Part model, mm, in its own coordinate system. Coordinates: 2 decimals unless noted, no trailing zeros. Write each loop counter-clockwise with the first axis right and the second up, starting at its lowest first coordinate (ties: lowest second). Pieces come first, ordered by that corner, then holes. Notation, with made-up numbers: (80, 5) -> (104, 5) arc R11 cw to (104, 11) -> close; hole circle Ø1 at (58, 56). An arc over 180 degrees is marked (long way). Write item = value, one per line.
from build123d import *

# Parameters (mm, degrees)
BOSS_EXTRUDE1_DEPTH      = 2.54
SKETCH2_W                = 0.64
SKETCH2_H                = 0.64
BOSS_EXTRUDE2_DEPTH      = 6
BOSS_EXTRUDE2_DEPTH_BACK = 5.74


with BuildPart() as part:
    # Sketch1 → Boss-Extrude1 (new body)
    with BuildSketch(Plane(origin=(0, 0, 0), x_dir=(1, 0, 0), z_dir=(0, 1, 0))):
        with BuildLine():
            Line((-11.43, -1.016), (-11.43, 1.016))
            ThreePointArc((-11.43, 1.016), (-11.504394878, 1.195605122), (-11.684, 1.27))
            Line((-11.684, 1.27), (-13.716, 1.27))
            ThreePointArc((-13.716, 1.27), (-13.895605122, 1.195605122), (-13.97, 1.016))
            Line((-13.97, 1.016), (-13.97, -1.016))
            ThreePointArc((-13.97, -1.016), (-13.895605122, -1.195605122), (-13.716, -1.27))
            Line((-13.716, -1.27), (-11.684, -1.27))
            ThreePointArc((-11.684, -1.27), (-11.504394878, -1.195605122), (-11.43, -1.016))
        make_face()
        with BuildLine():
            Line((-8.89, -1.016), (-8.89, 1.016))
            ThreePointArc((-8.89, 1.016), (-8.964394878, 1.195605122), (-9.144, 1.27))
            Line((-9.144, 1.27), (-11.176, 1.27))
            ThreePointArc((-11.176, 1.27), (-11.355605122, 1.195605122), (-11.43, 1.016))
            Line((-11.43, 1.016), (-11.43, -1.016))
            ThreePointArc((-11.43, -1.016), (-11.355605122, -1.195605122), (-11.176, -1.27))
            Line((-11.176, -1.27), (-9.144, -1.27))
            ThreePointArc((-9.144, -1.27), (-8.964394878, -1.195605122), (-8.89, -1.016))
        make_face()
        with BuildLine():
            Line((-6.35, -1.016), (-6.35, 1.016))
            ThreePointArc((-6.35, 1.016), (-6.424394878, 1.195605122), (-6.604, 1.27))
            Line((-6.604, 1.27), (-8.636, 1.27))
            ThreePointArc((-8.636, 1.27), (-8.815605122, 1.195605122), (-8.89, 1.016))
            Line((-8.89, 1.016), (-8.89, -1.016))
            ThreePointArc((-8.89, -1.016), (-8.815605122, -1.195605122), (-8.636, -1.27))
            Line((-8.636, -1.27), (-6.604, -1.27))
            ThreePointArc((-6.604, -1.27), (-6.424394878, -1.195605122), (-6.35, -1.016))
        make_face()
        with BuildLine():
            Line((-3.81, -1.016), (-3.81, 1.016))
            ThreePointArc((-3.81, 1.016), (-3.884394878, 1.195605122), (-4.064, 1.27))
            Line((-4.064, 1.27), (-6.096, 1.27))
            ThreePointArc((-6.096, 1.27), (-6.275605122, 1.195605122), (-6.35, 1.016))
            Line((-6.35, 1.016), (-6.35, -1.016))
            ThreePointArc((-6.35, -1.016), (-6.275605122, -1.195605122), (-6.096, -1.27))
            Line((-6.096, -1.27), (-4.064, -1.27))
            ThreePointArc((-4.064, -1.27), (-3.884394878, -1.195605122), (-3.81, -1.016))
        make_face()
        with BuildLine():
            Line((-1.27, -1.016), (-1.27, 1.016))
            ThreePointArc((-1.27, 1.016), (-1.344394878, 1.195605122), (-1.524, 1.27))
            Line((-1.524, 1.27), (-3.556, 1.27))
            ThreePointArc((-3.556, 1.27), (-3.735605122, 1.195605122), (-3.81, 1.016))
            Line((-3.81, 1.016), (-3.81, -1.016))
            ThreePointArc((-3.81, -1.016), (-3.735605122, -1.195605122), (-3.556, -1.27))
            Line((-3.556, -1.27), (-1.524, -1.27))
            ThreePointArc((-1.524, -1.27), (-1.344394878, -1.195605122), (-1.27, -1.016))
        make_face()
        with BuildLine():
            Line((1.27, -1.016), (1.27, 1.016))
            ThreePointArc((1.27, 1.016), (1.195605122, 1.195605122), (1.016, 1.27))
            Line((1.016, 1.27), (-1.016, 1.27))
            ThreePointArc((-1.016, 1.27), (-1.195605122, 1.195605122), (-1.27, 1.016))
            Line((-1.27, 1.016), (-1.27, -1.016))
            ThreePointArc((-1.27, -1.016), (-1.195605122, -1.195605122), (-1.016, -1.27))
            Line((-1.016, -1.27), (1.016, -1.27))
            ThreePointArc((1.016, -1.27), (1.195605122, -1.195605122), (1.27, -1.016))
        make_face()
        with BuildLine():
            Line((3.81, -1.016), (3.81, 1.016))
            ThreePointArc((3.81, 1.016), (3.735605122, 1.195605122), (3.556, 1.27))
            Line((3.556, 1.27), (1.524, 1.27))
            ThreePointArc((1.524, 1.27), (1.344394878, 1.195605122), (1.27, 1.016))
            Line((1.27, 1.016), (1.27, -1.016))
            ThreePointArc((1.27, -1.016), (1.344394878, -1.195605122), (1.524, -1.27))
            Line((1.524, -1.27), (3.556, -1.27))
            ThreePointArc((3.556, -1.27), (3.735605122, -1.195605122), (3.81, -1.016))
        make_face()
        with BuildLine():
            Line((6.35, -1.016), (6.35, 1.016))
            ThreePointArc((6.35, 1.016), (6.275605122, 1.195605122), (6.096, 1.27))
            Line((6.096, 1.27), (4.064, 1.27))
            ThreePointArc((4.064, 1.27), (3.884394878, 1.195605122), (3.81, 1.016))
            Line((3.81, 1.016), (3.81, -1.016))
            ThreePointArc((3.81, -1.016), (3.884394878, -1.195605122), (4.064, -1.27))
            Line((4.064, -1.27), (6.096, -1.27))
            ThreePointArc((6.096, -1.27), (6.275605122, -1.195605122), (6.35, -1.016))
        make_face()
        with BuildLine():
            Line((8.89, -1.016), (8.89, 1.016))
            ThreePointArc((8.89, 1.016), (8.815605122, 1.195605122), (8.636, 1.27))
            Line((8.636, 1.27), (6.604, 1.27))
            ThreePointArc((6.604, 1.27), (6.424394878, 1.195605122), (6.35, 1.016))
            Line((6.35, 1.016), (6.35, -1.016))
            ThreePointArc((6.35, -1.016), (6.424394878, -1.195605122), (6.604, -1.27))
            Line((6.604, -1.27), (8.636, -1.27))
            ThreePointArc((8.636, -1.27), (8.815605122, -1.195605122), (8.89, -1.016))
        make_face()
        with BuildLine():
            Line((11.43, -1.016), (11.43, 1.016))
            ThreePointArc((11.43, 1.016), (11.355605122, 1.195605122), (11.176, 1.27))
            Line((11.176, 1.27), (9.144, 1.27))
            ThreePointArc((9.144, 1.27), (8.964394878, 1.195605122), (8.89, 1.016))
            Line((8.89, 1.016), (8.89, -1.016))
            ThreePointArc((8.89, -1.016), (8.964394878, -1.195605122), (9.144, -1.27))
            Line((9.144, -1.27), (11.176, -1.27))
            ThreePointArc((11.176, -1.27), (11.355605122, -1.195605122), (11.43, -1.016))
        make_face()
        with BuildLine():
            Line((13.97, -1.016), (13.97, 1.016))
            ThreePointArc((13.97, 1.016), (13.895605122, 1.195605122), (13.716, 1.27))
            Line((13.716, 1.27), (11.684, 1.27))
            ThreePointArc((11.684, 1.27), (11.504394878, 1.195605122), (11.43, 1.016))
            Line((11.43, 1.016), (11.43, -1.016))
            ThreePointArc((11.43, -1.016), (11.504394878, -1.195605122), (11.684, -1.27))
            Line((11.684, -1.27), (13.716, -1.27))
            ThreePointArc((13.716, -1.27), (13.895605122, -1.195605122), (13.97, -1.016))
        make_face()
    extrude(amount=BOSS_EXTRUDE1_DEPTH)

    # Sketch2 → Boss-Extrude2 (add, two sides)
    with BuildSketch(Plane(origin=(0, 2.54, 0), x_dir=(1, 0, 0), z_dir=(0, 1, 0))) as boss_extrude2_sk:
        with Locations((-12.7, 0)):
            Rectangle(SKETCH2_W, SKETCH2_H)
        with Locations((-10.16, 0)):
            Rectangle(SKETCH2_W, SKETCH2_H)
        with Locations((-7.62, 0)):
            Rectangle(SKETCH2_W, SKETCH2_H)
        with Locations((-5.08, 0)):
            Rectangle(SKETCH2_W, SKETCH2_H)
        with Locations((-2.54, 0)):
            Rectangle(SKETCH2_W, SKETCH2_H)
        Rectangle(SKETCH2_W, SKETCH2_H)
        with Locations((2.54, 0)):
            Rectangle(SKETCH2_W, SKETCH2_H)
        with Locations((5.08, 0)):
            Rectangle(SKETCH2_W, SKETCH2_H)
        with Locations((7.62, 0)):
            Rectangle(SKETCH2_W, SKETCH2_H)
        with Locations((10.16, 0)):
            Rectangle(SKETCH2_W, SKETCH2_H)
        with Locations((12.7, 0)):
            Rectangle(SKETCH2_W, SKETCH2_H)
    extrude(amount=BOSS_EXTRUDE2_DEPTH)
    extrude(boss_extrude2_sk.sketch, amount=-BOSS_EXTRUDE2_DEPTH_BACK)


solid = part.part
Q1. Saw through at A-A on y = 5. Count the separate pieces of the cut face and the enclosed holes in it, and give its area (3 significant figures).
Model answer:
separate_pieces = 11
enclosed_holes = 0
area = 4.51 mm²
Q2. Probe line 1 (Y direction, x = -2, z = 0.85); line 2 (Z direction, x = 0.25, y = 3.5). List the from-to ranges inside material, lowest first. Write a range as from..to.
Model answer:
line_1 = 0..2.54
line_2 = -0.32..0.32
Q3. Mould opens along X. For faces 1 (the face through (0, 0, -1)), 2 (the face through (13.97, 1, 0)), 3 (the face through (0, 2.54, -1)), 4 (the face through (8, 1, 1.27)) say: released by +X, released by -X, zero draft, split by the parting line, or undercut.
Model answer:
face_1 = undercut
face_2 = released by +X
face_3 = undercut
face_4 = zero draft
Q4. Pin check, flat tips, straight feed: pin 1 (0.7 mm diameter, centred on y = 5, z = 0, fed in from -X); pin 2 (0.5 mm diameter, centred on y = 7, z = 0, fed in from +X); pin 3 (0.5 mm diameter, centred on x = 0, y = 5, fed in from -Z). Stop position of each tip, or through.
Model answer:
pin_1 = -13.02
pin_2 = 13.02
pin_3 = -0.32
Q5. Saw through at B-B on x = 2.5. Give the cut face in (y, z), and give its area (3 significant figures).
Model answer:
outline = (-3.2, -0.32) -> (0, -0.32) -> (0, -1.27) -> (2.54, -1.27) -> (2.54, -0.32) -> (8.54, -0.32) -> (8.54, 0.32) -> (2.54, 0.32) -> (2.54, 1.27) -> (0, 1.27) -> (0, 0.32) -> (-3.2, 0.32) -> close
area = 12.3 mm²
Q6. Saw through at D-D on x = -10.75. Give the cut face in (y, z), and give its area (3 significant figures).
Model answer:
outline = (0, -1.27) -> (2.54, -1.27) -> (2.54, 1.27) -> (0, 1.27) -> close
area = 6.45 mm²
Q7. Saw through at C-C on z = -0.65. Give the cut face in (x, y), and give its area (3 significant figures).
Model answer:
outline = (-13.97, 0) -> (13.97, 0) -> (13.97, 2.54) -> (-13.97, 2.54) -> close
area = 71.0 mm²
